For this review, take the finished solid that the model builds, in its own axes (mm). A direction names the side the tool comes from. Coordinates: 2 decimals unless noted, no trailing zeros. Loops run counter-clockwise (first coordinate to the right, second up) from the corner with the lowest first, then second, coordinate; pieces in that order, holes last.
```python
from build123d import *

# Parameters (mm, degrees)
F0_W     = 596.9
F0_H     = 762
F0_W_2   = 558.8
F0_H_2   = 723.9
F1_DEPTH = 152.4
F2_W     = 6.35
F2_H     = 6.35
F3_DEPTH = 723.9


with BuildPart() as f1:
    # F0 (on Front) → F1 (new body)
    with BuildSketch(Plane.XZ):
        with Locations((-279.4, 361.95)):
            Rectangle(F0_W, F0_H)
        with Locations((-279.4, 361.95)):
            Rectangle(F0_W_2, F0_H_2, mode=Mode.SUBTRACT)
    extrude(amount=F1_DEPTH)

    # F2 (on face) → F3 (join, through all)
    with BuildSketch(Plane.XY):
        with Locations((-555.625, -79.375)):
            Rectangle(F2_W, F2_H)
        with Locations((-3.175, -79.375)):
            Rectangle(F2_W, F2_H)
    extrude(amount=F3_DEPTH)


solid = f1.part
```
Q1. Consider section B-B (y = -66.5). State the section outline as (x, z) points.
Q2. Consider section C-C (x = -210). State the section outline as (y, z) points, then the cut area to 3 significant figures.
Q3. For pin 1 Ø5 at (x, z) = (-555.5, 425.5) entering from +Y; pin 2 Ø7 at (x, z) = (-4, 417.5) entering from -Y, all flat-tipped, find the tip position at first contact; note any pin that passes through.
Q4. Consider section A-A (z = 562.5). State the section outline as (x, y) points, then the cut area to 3 significant figures.
Q5. Machinability: for faces 1 (the face through (-558.8, -38, 357)), 2 (the face through (-568, 0, 364)), 3 (the face through (-558.8, -117, 357)), which of the approach directions +Z, -Z, +X, -X, +Y, -Y give a long, thin tool a straight path to every point of the face, cutting with its end or side? Answer none if there is none.
Q6. The part is to be moulded in two halves that separate along X. For faces 4 (the face through (-568, -152.4, 364)), 5 (the face through (0, -38, 357)), 6 (the face through (-577.85, -75, 357)), say which applies: +X half, -X half, draft (parallel to the pull), parting line (faces both ways), or undercut.
Q7. Wall thickness on probe 1 along X at (y, z) = (-8, 382); probe 2 along Z at (x, y) = (-539, -66): over which ranges is each line inside the solid? List them lowest first.
Model answer:
1. outline: (-577.85, -19.05) - (19.05, -19.05) - (19.05, 742.95) - (-577.85, 742.95) - close; hole (-558.8, 0) - (0, 0) - (0, 723.9) - (-558.8, 723.9) - close
2. outline: (-152.4, -19.05) - (0, -19.05) - (0, 0) - (-152.4, 0) - close; (-152.4, 723.9) - (0, 723.9) - (0, 742.95) - (-152.4, 742.95) - close
2. area: 5,810 mm2
3. pin 1: stops at y = -76.2
3. pin 2: stops at y = -82.55
4. outline: (-577.85, -152.4) - (-558.8, -152.4) - (-558.8, -82.55) - (-552.45, -82.55) - (-552.45, -76.2) - (-558.8, -76.2) - (-558.8, 0) - (-577.85, 0) - close; (-6.35, -82.55) - (0, -82.55) - (0, -152.4) - (19.05, -152.4) - (19.05, 0) - (0, 0) - (0, -76.2) - (-6.35, -76.2) - close
4. area: 5,890 mm2
5. face 1: +Y
5. face 2: +Z, -Z, +X, -X, +Y
5. face 3: -Y
6. face 4: draft
6. face 5: undercut
6. face 6: -X half
7. probe 1: x = -577.85 to -558.8, 0 to 19.05
7. probe 2: z = -19.05 to 0, 723.9 to 742.95
